The listing builds one solid part. Answer for the finished solid, in the listing's coordinates (mm). Give positions to 0.01 mm unless a question says otherwise; leave off trailing zeros. Order: outer loops, then holes, each group sorted by start corner. A loop starts at its lowest first (then second) coordinate and runs counter-clockwise, first axis right, second up. Notation, with made-up numbers: (7, 37) - (60, 37) arc R18 cw to (60, 44) - close; hole circle Ø11 at (63.25, 17). An arc over 180 degrees is marked (long way). Write each question's results on one line, items separated by ' | '. Start each with the question number.
1. Flat-ended cylindrical pins translate along their axes: pin 1 (15 mm diameter, centred on x = 85.37, z = 20.31, fed in from +Y); pin 2 (1 mm diameter, centred on y = -2, z = 84, fed in from +X). Find the tip coordinate at first contact, or state that the pin passes through.
2. Find the intervals of material crossed by L1, parallel to Z at x = 10, y = -2.7; L2, parallel to Z at x = 7.5, y = -3.5; L3, parallel to X at y = -0.95, z = 30, in increasing order.
3. Section B-B (x = 10) is taken. Give the vertices of the cut face in (y, z), and give its area (3 significant figures).
4. Determine the mould class of faces 1 (the face through (100, -2, 15)), 2 (the face through (12.77, -1.97, 11.35)), 3 (the face through (9.609, -1.972, 61.828)), 4 (the face through (40, -4, 38)) for opening direction X: released by +X, released by -X, zero draft, split by the parting line, or undercut.
5. Section A-A (z = 20.31) is taken. Give the vertices of the cut face in (x, y).
6. Section C-C (x = 83.5) is taken. Give the vertices of the cut face in (y, z), and give its area (3 significant figures).
7. Section D-D (y = -1.6) is taken. Give the vertices of the cut face in (x, z), and give its area (3 significant figures).
Solid Edge part; units mm, degrees
sketch "Sketch1" plane through (0, 0, 0) normal (0, -1, 0) x (1, 0, 0)
  circle A0 centre (10, 10.2) radius 3
  circle A1 centre (85.37, 20.31) radius 6.45
  circle A2 centre (10, 30.2) radius 3
  line L0 (24.0066, 95) -> (0, 95)
  line L1 (0, 95) -> (0, 0)
  line L2 (0, 0) -> (100, 0)
  line L3 (100, 0) -> (100, 30)
  line L4 (100, 30) -> (24.0066, 95)
  circle A3 centre (10, 84.802) radius 3
  circle A4 centre (10, 64.802) radius 3
extrude "Protrusion1" add sketch "Sketch1" along normal blind 4
Reported:
1) pin 1: y = 0 | pin 2: x = 37.45
2) L1: 0 to 7.2, 13.2 to 27.2, 33.2 to 61.8, 67.8 to 81.8, 87.8 to 95 | L2: 0 to 8.54, 11.86 to 28.54, 31.86 to 63.14, 66.46 to 83.14, 86.46 to 95 | L3: 0 to 7.01, 12.99 to 100
3) outline: (-4, 0) - (0, 0) - (0, 7.2) - (-4, 7.2) - close; (-4, 13.2) - (0, 13.2) - (0, 27.2) - (-4, 27.2) - close; (-4, 33.2) - (0, 33.2) - (0, 61.8) - (-4, 61.8) - close; (-4, 67.8) - (0, 67.8) - (0, 81.8) - (-4, 81.8) - close; (-4, 87.8) - (0, 87.8) - (0, 95) - (-4, 95) - close | area: 284 mm²
4) face 1: released by +X | face 2: undercut | face 3: undercut | face 4: zero draft
5) outline: (0, -4) - (78.92, -4) - (78.92, 0) - (0, 0) - close; (91.82, -4) - (100, -4) - (100, 0) - (91.82, 0) - close
6) outline: (-4, 0) - (0, 0) - (0, 14.14) - (-4, 14.14) - close; (-4, 26.48) - (0, 26.48) - (0, 44.11) - (-4, 44.11) - close | area: 127 mm²
7) outline: (0, 0) - (100, 0) - (100, 30) - (24.01, 95) - (0, 95) - close; hole circle Ø6 at (10, 10.2); hole circle Ø6 at (10, 30.2); hole circle Ø6 at (10, 64.8); hole circle Ø6 at (10, 84.8); hole circle Ø12.9 at (85.37, 20.31) | area: 6,790 mm²
